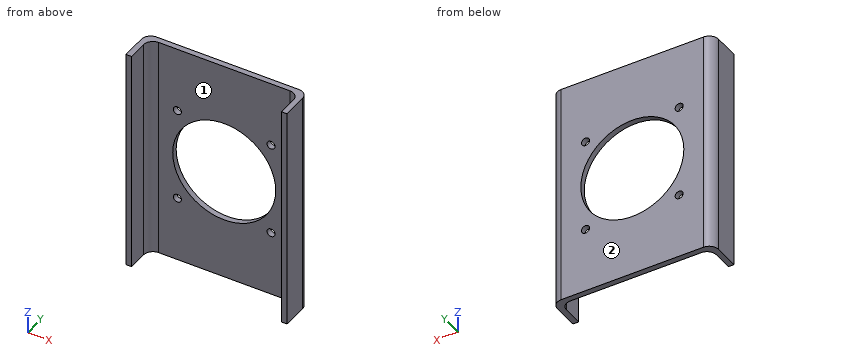
Autodesk Inventor part; units mm, degrees
ref_plane "YZ Plane" through (0, 0, 0) normal (1, 0, 0) x (0, 1, 0)
ref_plane "XZ Plane" through (0, 0, 0) normal (0, 1, 0) x (-1, 0, 0)
ref_plane "XY Plane" through (0, 0, 0) normal (0, 0, 1) x (1, 0, 0)
sketch "Sketch1" plane through (0, 0, 0) normal (0, 0, 1) x (1, 0, 0)
  line L0 (0, 0) -> (40, 0)
  line L1 (0, 0) -> (0, -20) construction
  line L2 (40, 0) -> (40, -15.5)
  line L3 (0, 0) -> (40, 0)
  line L4 (40, 0) -> (40, 3)
  line L5 (40, 3) -> (0, 3)
  line L6 (0, 3) -> (0, 0)
  line L7 (40, 3) -> (43, 3)
  line L8 (43, 3) -> (43, -15.5)
  line L9 (43, -15.5) -> (40, -15.5)
  line L10 (40, -15.5) -> (40, 3)
  line L11 (0, 0) -> (-40, 0)
  line L12 (-40, 0) -> (-40, -15.5)
  line L13 (-40, 3) -> (0, 3)
  line L14 (-40, 3) -> (-43, 3)
  line L15 (-43, 3) -> (-43, -15.5)
  line L16 (-43, -15.5) -> (-40, -15.5)
  point P0 (41.5, -15.5)
  dimension "d0" = 40
  dimension "d1" = 20
  dimension "d3" = 3
  dimension "d4" = 3
  dimension "d17" = 15.5
extrude "Extrusion1" add sketch "Sketch1" along normal blind 120
sketch "Sketch2" plane through (-43, 3, 0) normal (0, 1, 0) x (1, 0, 0)
  line L0 (86, 0) -> (86, -120)
  line L1 (86, -60) -> (0, -60) construction
  line L2 (0, 0) -> (0, -120)
  line L3 (68, -35) -> (18, -35) construction
  line L4 (18, -35) -> (18, -85) construction
  line L5 (18, -85) -> (68, -85) construction
  line L6 (68, -85) -> (68, -35) construction
  line L7 (68, -35) -> (18, -85) construction
  line L8 (18, -35) -> (68, -85) construction
  circle A0 centre (68, -85) radius 2.15
  circle A1 centre (18, -85) radius 2.15
  circle A2 centre (68, -35) radius 2.15
  circle A3 centre (18, -35) radius 2.15
  circle A4 centre (43, -60) radius 27.5
  point P0 (43, 0)
  dimension "d7" = 50
  dimension "d8" = 50
  dimension "d9" = 4.3
  dimension "d10" = 4.3
  dimension "d11" = 4.3
  dimension "d12" = 4.3
  dimension "d15" = 55
extrude "Extrusion2" cut sketch "Sketch2" against normal through all
fillet "Fillet1" radius 5 4 edges at (40, 0, 60) (43, 3, 60) (-40, 0, 60) (-43, 3, 60)
properties part number "FanHolder"
Input: part model. Units: mm. Frame: model coordinates. Face numbers are marked on the shaded views. Give positions to 0.01 mm unless a question says otherwise; leave off trailing zeros. Order: outer loops, then holes, each group sorted by start corner. A loop starts at its lowest first (then second) coordinate and runs counter-clockwise, first axis right, second up. Notation, with made-up numbers: (29.25, -23.75) - (48.25, -23.75) arc R12 cw to (48.25, -7.75) - close; hole circle Ø9 at (-17, 21). An arc over 180 degrees is marked (long way). One line per item, written item: value.
1. Cut plane D-D, the plane z = 93. Output: boundary loops of the cut face in (x, y).
Determined:
outline: (-43, -15.5) - (-40, -15.5) - (-40, -5) arc R5 cw to (-35, 0) - (35, 0) arc R5 cw to (40, -5) - (40, -15.5) - (43, -15.5) - (43, -2) arc R5 ccw to (38, 3) - (-38, 3) arc R5 ccw to (-43, -2) - close
2. Cut plane C-C, the plane x = 25. Output: boundary loops of the cut face in (y, z), and give its area (3 significant figures).
Determined:
outline: (0, 0) - (3, 0) - (3, 32.85) - (0, 32.85) - close; (0, 37.15) - (3, 37.15) - (3, 48.54) - (0, 48.54) - close; (0, 71.46) - (3, 71.46) - (3, 82.85) - (0, 82.85) - close; (0, 87.15) - (3, 87.15) - (3, 120) - (0, 120) - close
area: 265 mm2
3. Draft query along Y for the marked faces 1 and 2. Return one class per face: released by +Y, released by -Y, zero draft, split by the parting line, or undercut.
Determined:
face 1: released by -Y
face 2: released by +Y
4. Cut plane B-B, the plane z = 60. Output: boundary loops of the cut face in (x, y).
Determined:
outline: (-43, -15.5) - (-40, -15.5) - (-40, -5) arc R5 cw to (-35, 0) - (-27.5, 0) - (-27.5, 3) - (-38, 3) arc R5 ccw to (-43, -2) - close; (27.5, 0) - (35, 0) arc R5 cw to (40, -5) - (40, -15.5) - (43, -15.5) - (43, -2) arc R5 ccw to (38, 3) - (27.5, 3) - close
5. Line query: probe 1 along X at (y, z) = (-10.75, 96); probe 2 along Z at (x, y) = (25, 1.85); probe 3 along X at (y, z) = (1.25, 35). Output: solid intervals per line, ascending.
Determined:
probe 1: -43 to -40, 40 to 43
probe 2: 0 to 32.85, 37.15 to 48.54, 71.46 to 82.85, 87.15 to 120
probe 3: -41.8 to -27.15, -22.85 to -11.46, 11.46 to 22.85, 27.15 to 41.8
6. Cut plane A-A, the plane y = -9.25. Output: boundary loops of the cut face in (x, z), and give its area (3 significant figures).
Determined:
outline: (-43, 0) - (-40, 0) - (-40, 120) - (-43, 120) - close; (40, 0) - (43, 0) - (43, 120) - (40, 120) - close
area: 720 mm2
7. Pin query (flat end, axial travel): pin 1 Ø1 at (x, z) = (1.5, 97.5) entering from -Y. Return the tip coordinate at first contact, or that it passes through.
Determined:
pin 1: y = 0
